from build123d import *

# Parameters (mm, degrees)
CHANFREIN1_SIZE              = 0.5
BOSS_EXTRU_1_START           = 5.5
BOSS_EXTRU_1_DEPTH           = 5.5
BOSS_EXTRU_2_START           = -3.6
BOSS_EXTRU_2_DEPTH           = 3.6
R_P_TITION_CIRCULAIRE1_COUNT = 2


with BuildPart() as part:
    # Esquisse1 → Révolution1 (revolve)
    with BuildSketch(Plane.XY, mode=Mode.PRIVATE) as r_volution1_sk:
        with BuildLine():
            Line((0, 0), (0, 46.75))
            Line((0, 46.75), (5.5, 46.75))
            Line((5.5, 46.75), (5.5, 48.5))
            Line((5.5, 48.5), (2.5, 48.5))
            Line((2.5, 48.5), (2.5, 50))
            Line((2.5, 50), (-2.5, 50))
            ThreePointArc((-2.5, 50), (-3.914213562, 49.414213562), (-4.5, 48))
            Line((-4.5, 48), (-4.5, 0))
            Line((-4.5, 0), (0, 0))
        make_face()
    revolve(r_volution1_sk.sketch.rotate(Axis((0, 0, 0), (-1, 0, 0)), 90), axis=Axis((0, 0, 0), (-1, 0, 0)))

    # Chanfrein1
    chanfrein1_edges = [part.edges().sort_by_distance(p)[0] for p in [
        (5.5, 0, 48.5),
    ]]
    chamfer(chanfrein1_edges, length=CHANFREIN1_SIZE)

    # Esquisse2 → Boss.-Extru.1 (add)
    with BuildSketch(Plane(origin=(0, 0, 0), x_dir=(0, 0, -1), z_dir=(1, 0, 0)).offset(BOSS_EXTRU_1_START)):
        with BuildLine():
            Line((-10, 45.667959227), (-10, 28.5))
            Line((-10, 28.5), (10, 28.5))
            Line((10, 28.5), (10, 45.667959227))
            ThreePointArc((10, 45.667959227), (0, 46.75), (-10, 45.667959227))
        make_face()
        with BuildLine():
            Line((-10, -28.5), (10, -28.5))
            Line((10, -28.5), (10, -45.667959227))
            ThreePointArc((10, -45.667959227), (0, -46.75), (-10, -45.667959227))
            Line((-10, -45.667959227), (-10, -28.5))
        make_face()
    extrude(amount=-BOSS_EXTRU_1_DEPTH)

    # Esquisse3 → Boss.-Extru.2 (add)
    with BuildSketch(Plane(origin=(2.5, 0, 0), x_dir=(0, 0, -1), z_dir=(1, 0, 0)).offset(BOSS_EXTRU_2_START)):
        with BuildLine():
            Line((-8, 54.5), (-8, 49.355850717))
            ThreePointArc((-8, 49.355850717), (0, 50), (8, 49.355850717))
            Line((8, 49.355850717), (8, 54.5))
            ThreePointArc((8, 54.5), (7.707106781, 55.207106781), (7, 55.5))
            Line((7, 55.5), (5.5, 55.5))
            ThreePointArc((5.5, 55.5), (0, 55), (-5.5, 55.5))
            Line((-5.5, 55.5), (-7, 55.5))
            ThreePointArc((-7, 55.5), (-7.707106781, 55.207106781), (-8, 54.5))
        make_face()
    boss_extru_2 = extrude(amount=BOSS_EXTRU_2_DEPTH)

    # Répétition circulaire1: Boss.-Extru.2 ×2 about axis
    r_p_tition_circulaire1_axis = Axis((0, 0, 0), (1, 0, 0))
    for i in range(1, R_P_TITION_CIRCULAIRE1_COUNT):
        add(boss_extru_2.rotate(r_p_tition_circulaire1_axis, i * 360 / R_P_TITION_CIRCULAIRE1_COUNT))


solid = part.part
Build history of the part. All positions in model axes, mm. A direction names the side the tool comes from. Coordinates: 2 decimals unless noted, no trailing zeros. Write each loop counter-clockwise with the first axis right and the second up, starting at its lowest first coordinate (ties: lowest second). Pieces come first, ordered by that corner, then holes.
(1) 3-axis set-ups, long thin cutter, end or side, ignore diameter. For faces 5 (the flat face through (1, 52, -8)), 6 (the flat face through (3, -37, -10)), 7 (the flat face through (5.5, -29, 0)), 8 (the flat face through (1, -52, -8)), 9 (the flat face through (1, 52, 8)): which of +Z, -Z, +X, -X, +Y, -Y reach the whole face in a straight line?
(2) Cut at A-A on y = 0. List the corners of the cut face in (x, z).
(3) Pin check, flat tips, straight feed: pin 1 Ø6 at (y, z) = (36, -20.5) entering from +X; pin 2 Ø1.6 at (x, z) = (3.5, 3.5) entering from +Y; pin 3 Ø4 at (x, z) = (2.5, 29.5) entering from +Y. Stop position of each tip, or through.
(4) Cut at B-B on z = 0. List the corners of the cut face in (x, y).
(5) Mould opens along Y. For faces 1 (the flat face through (3, -37, 10)), 2 (the flat face through (-4.5, -1, 1)), 3 (the cylindrical face through (3.732, 43.028, -22.38)), 4 (the flat face through (3, 37, 10)) say: pulls with the +Y half, pulls with the -Y half, needs draft (parallel to the pull), parting line crosses it, or undercut.
(6) Drill centre lines: line 1 (Z direction, x = 0.75, y = 39); line 2 (Z direction, x = 4, y = 40); line 3 (Y direction, x = 4.75, z = -35.5). Where is each one in solid material? Low to high.
Working result:
1. face 5: -Z, +X, -X, +Y
1. face 6: +X
1. face 7: +Z, -Z, +X, +Y, -Y
1. face 8: -Z, +X, -X, -Y
1. face 9: +Z, +X, -X, +Y
2. outline: (-4.5, -48) arc R2 ccw to (-2.5, -50) - (2.5, -50) - (2.5, -48.5) - (5, -48.5) - (5.5, -48) - (5.5, -46.75) - (0, -46.75) - (0, 46.75) - (5.5, 46.75) - (5.5, 48) - (5, 48.5) - (2.5, 48.5) - (2.5, 50) - (-2.5, 50) arc R2 ccw to (-4.5, 48) - close
3. pin 1: stops at x = 0
3. pin 2: stops at y = 48.42
3. pin 3: stops at y = 41.76
4. outline: (-4.5, -48) arc R2 ccw to (-2.5, -50) - (-1.1, -50) - (-1.1, -55) - (2.5, -55) - (2.5, -48.5) - (5, -48.5) - (5.5, -48) - (5.5, -28.5) - (0, -28.5) - (0, 28.5) - (5.5, 28.5) - (5.5, 48) - (5, 48.5) - (2.5, 48.5) - (2.5, 55) - (-1.1, 55) - (-1.1, 50) - (-2.5, 50) arc R2 ccw to (-4.5, 48) - close
5. face 1: undercut
5. face 2: needs draft
5. face 3: parting line crosses it
5. face 4: undercut
6. line 1: z = -31.29 to -25.78, -10 to 10, 25.78 to 31.29
6. line 2: z = -27.43 to -24.2, -10 to 10, 24.2 to 27.43
6. line 3: y = -33.05 to -30.42, 30.42 to 33.05
